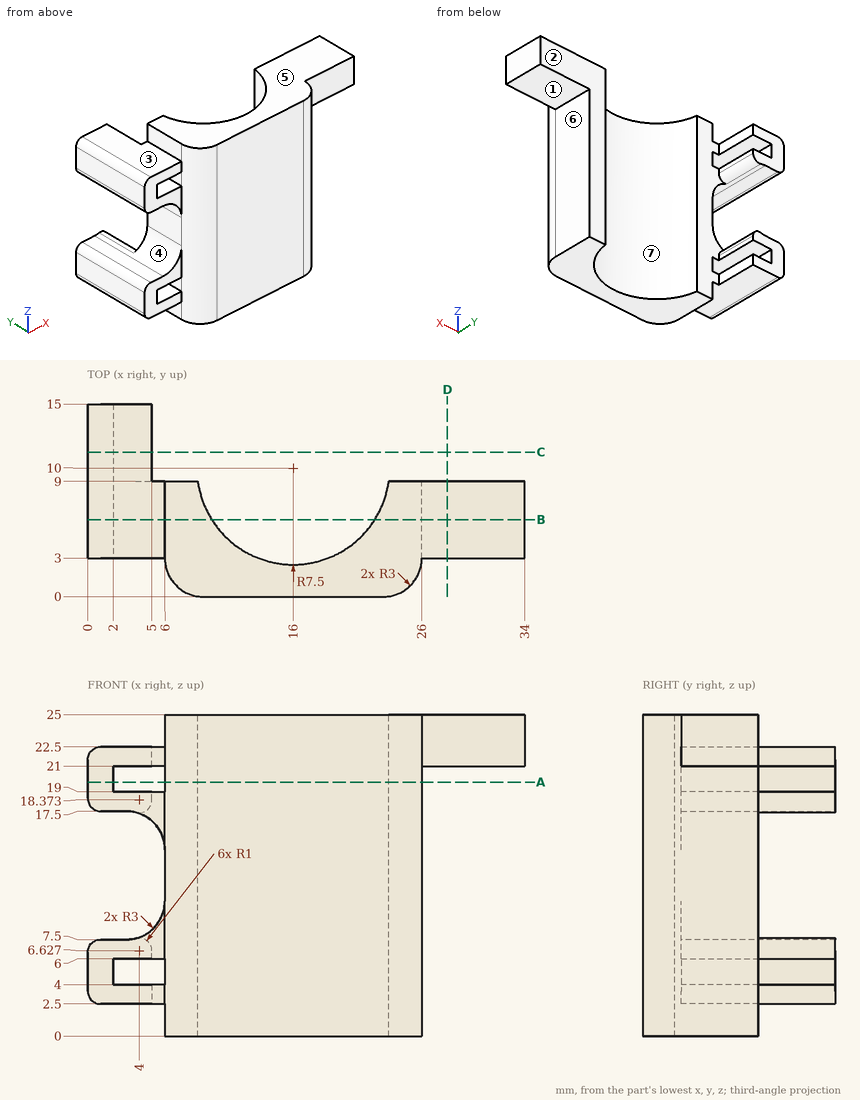
The figure shows three views and two pictorial views of one solid part (mm, origin at its lowest corner). Answer the questions. A direction names the side the tool comes from. Coordinates: 2 decimals unless noted, no trailing zeros. Loops run counter-clockwise (first coordinate to the right, second up) from the corner with the lowest first, then second, coordinate; pieces in that order, holes last.
1) Determine the mould class of the marked faces 5, 6 and 7 for opening direction X: pulls with the +X half, pulls with the -X half, needs draft (parallel to the pull), parting line crosses it, or undercut.
2) Find the intervals of material crossed by L1, parallel to X at y = 4.25, z = 5; L2, parallel to Z at x = 4, y = 5.5; L3, parallel to X at y = 5.25, z = 13, in increasing order.
3) Find section A-A on z = 19.75. Write down the section's boundary in (x, y), then the cut area to 3 significant figures.
4) Find section B-B on y = 6. Give the number of separate pieces and of enclosed holes in the cut face, then the cut area to 3 significant figures.
5) A tool of negligible diameter and unlimited length cuts with its end or side. For the marked faces 1, 2, 3 and 4, from which of +Z, -Z, +X, -X, +Y, -Y can it reach the whole face along a straight path? Write none if from no direction.
6) Flat-ended cylindrical pins translate along their axes: pin 1 Ø1.8 at (x, z) = (2, 4.5) entering from -Y; pin 2 Ø3 at (x, z) = (28, 12) entering from +Y; pin 3 Ø6.5 at (x, z) = (4, 19.5) entering from -Y; pin 4 Ø1 at (y, z) = (7, 4.5) entering from +X. Find the tip coordinate at first contact, or state that the pin passes through.
7) Find section C-C on y = 11.25. Write down the section's boundary in (x, z).
8) Find section D-D on x = 28. Write down the section's boundary in (y, z), then the cut area to 3 significant figures.
Values:
1. face 5: needs draft
1. face 6: pulls with the +X half
1. face 7: undercut
2. L1: x = 0 to 2, 6 to 11.18, 20.82 to 26
2. L2: z = 2.5 to 4, 6 to 7.67, 17.33 to 19, 21 to 22.5
2. L3: x = 6 to 10.2, 21.8 to 26
3. outline: (0, 3) - (2, 3) - (2, 15) - (0, 15) - close; (6, 3) arc R3 ccw to (9, 0) - (23, 0) arc R3 ccw to (26, 3) - (26, 9) - (23.43, 9) arc R7.5 cw to (8.57, 9) - (6, 9) - close
3. area: 127 mm2
4. separate pieces: 2
4. enclosed holes: 2
4. area: 262 mm2
5. face 1: -Z, +X, +Y, -Y
5. face 2: +Z, -Z, +X, +Y
5. face 3: +Z, -X, +Y, -Y
5. face 4: -X, +Y, -Y
6. pin 1: stops at y = 3
6. pin 2: passes through
6. pin 3: stops at y = 0.56
6. pin 4: stops at x = 26
7. outline: (0, 3.5) arc R1 ccw to (1, 2.5) - (5, 2.5) - (5, 4) - (2, 4) - (2, 6) - (5, 6) - (5, 6.63) arc R1 ccw to (3.75, 7.6) arc R3 cw to (3, 7.5) - (1, 7.5) arc R1 ccw to (0, 6.5) - close; (0, 18.5) arc R1 ccw to (1, 17.5) - (3, 17.5) arc R3 cw to (3.75, 17.4) arc R1 ccw to (5, 18.37) - (5, 19) - (2, 19) - (2, 21) - (5, 21) - (5, 22.5) - (1, 22.5) arc R1 ccw to (0, 21.5) - close
8. outline: (3, 21) - (9, 21) - (9, 25) - (3, 25) - close
8. area: 24.0 mm2
